For this review, take the finished solid that the model builds, in its own axes (mm). A direction names the side the tool comes from. Coordinates: 2 decimals unless noted, no trailing zeros. Write each loop counter-clockwise with the first axis right and the second up, starting at its lowest first coordinate (ties: lowest second). Pieces come first, ordered by that corner, then holes. Notation, with made-up numbers: (86, 44.25) - (97, 44.25) arc R29 cw to (97, 71.25) - close; hole circle Ø7 at (33.25, -33). An arc over 180 degrees is marked (long way). Use one line per item in the form item = value. Start each with the question number.
1) For L1, parallel to Y at x = 11, z = 1.75; L2, parallel to X at y = 35.5, z = 19.5; L3, parallel to Y at x = 8, z = 19, list the stretches that pass through material, from the lowest coordinate up. Write a range as from..to.
2) Mouldability with a two-part tool opening along X and no side actions: class faces 3 (the flat face through (0, -10, 25.4)), 4 (the cylindrical face through (-2.45, 36.43, 12.52)), 5 (the flat face through (2.57, -41.72, 12.52)) as pulls with the +X half, pulls with the -X half, needs draft (parallel to the pull), parting line crosses it, or undercut.
3) We need section C-C (y = 22). Give the boundary of the cut face in (x, z).
4) Tool access review of faces 1 (the flat face through (19.93, -2.75, 12.52)), 2 (the flat face through (22.498, -27.25, 12.522)): name each direction out of +Z, -Z, +X, -X, +Y, -Y from which nothing blocks a thin tool from reaching the whole face with its end or side.
5) Insertion check: P1, Ø13, axis at x = -5.18, y = 32.16, coming from the +Z side; P2, Ø1.5, axis at x = 0.5, z = 8.5, coming from the -Y side; P3, Ø10, axis at y = -0.5, z = 13.5, coming from the +X side; P4, Ø4, axis at x = 9, z = 18, coming from the -Y side. Each pin has a flat end and moves straight along its axis. Give the tip position at first contact, or say it passes through.
6) We need section B-B (x = -24). Give the boundary of the cut face in (y, z).
7) We need section A-A (z = 7.25). Give the boundary of the cut face in (x, y), plus the area to 3 significant figures.
```python
from build123d import *

# Parameters (mm, degrees)
F0_R     = 5.0729517485
F0_R_2   = 5.2620851013
F1_DEPTH = 25.4


with BuildPart() as f1:
    # F0 (on Top) → F1 (new body)
    with BuildSketch(Plane.XY):
        with BuildLine():
            ThreePointArc((6.3195106697, 8.2748654283), (14.1949379045, 14.5853247175), (17.1620698292, 24.23106879))
            ThreePointArc((17.1620698292, 24.23106879), (-11.1785461031, 37.2532325059), (-2.5997362388, 7.2670476773))
            Line((-2.5997362388, 7.2670476773), (6.3195106697, 8.2748654283))
        make_face()
        with Locations((-5.181599874, 32.1565270424)):
            Circle(F0_R, mode=Mode.SUBTRACT)
        with Locations((6.4008007757, 32.1565270424)):
            Circle(F0_R_2, mode=Mode.SUBTRACT)
        with BuildLine():
            Line((6.3195106697, 8.2748654283), (-2.5997362388, 7.2670476773))
            ThreePointArc((-2.5997362388, 7.2670476773), (1.9269417763, 7.1775197102), (6.3195106697, 8.2748654283))
        make_face()
        with BuildLine():
            ThreePointArc((6.3195106697, 8.2748654283), (1.9269417763, 7.1775197102), (-2.5997362388, 7.2670476773))
            Line((-2.5997362388, 7.2670476773), (-16.8951326659, 5.651759478))
            Line((-16.8951326659, 5.651759478), (-28.2595672484, -20.4183186727))
            Line((-28.2595672484, -20.4183186727), (-11.3644345824, -43.2952467961))
            Line((-11.3644345824, -43.2952467961), (16.8951326659, -40.1020967688))
            Line((16.8951326659, -40.1020967688), (28.2595672484, -14.0320186181))
            Line((28.2595672484, -14.0320186181), (11.3644345824, 8.8449095053))
            Line((11.3644345824, 8.8449095053), (6.3195106697, 8.2748654283))
        make_face()
    extrude(amount=F1_DEPTH)


solid = f1.part
```
Determined:
q1.L1 = -40.77..8.8, 11.06..29.6, 34.71..37.4
q1.L2 = -12.94..-9, -1.37..2.34, 10.46..12.94
q1.L3 = -41.11..8.46, 9.05..27.14, 37.17..39.41
q2.face_3 = needs draft
q2.face_4 = undercut
q2.face_5 = pulls with the +X half
q3.outline = (-17.02, 0) - (17.02, 0) - (17.02, 25.4) - (-17.02, 25.4) - close
q4.face_1 = +Z, -Z, +X
q4.face_2 = +Z, -Z, +X, -Y
q5.P1 = 25.4
q5.P2 = -42.04
q5.P3 = 21.96
q5.P4 = -41.22
q6.outline = (-26.19, 0) - (-10.65, 0) - (-10.65, 25.4) - (-26.19, 25.4) - close
q7.outline = (-28.26, -20.42) - (-11.36, -43.3) - (16.9, -40.1) - (28.26, -14.03) - (11.36, 8.84) - (6.32, 8.27) arc R17.16 ccw (long way) to (-2.6, 7.27) - (-16.9, 5.65) - close; hole circle Ø10.15 at (-5.18, 32.16); hole circle Ø10.52 at (6.4, 32.16)
q7.area = 2,860 mm²
